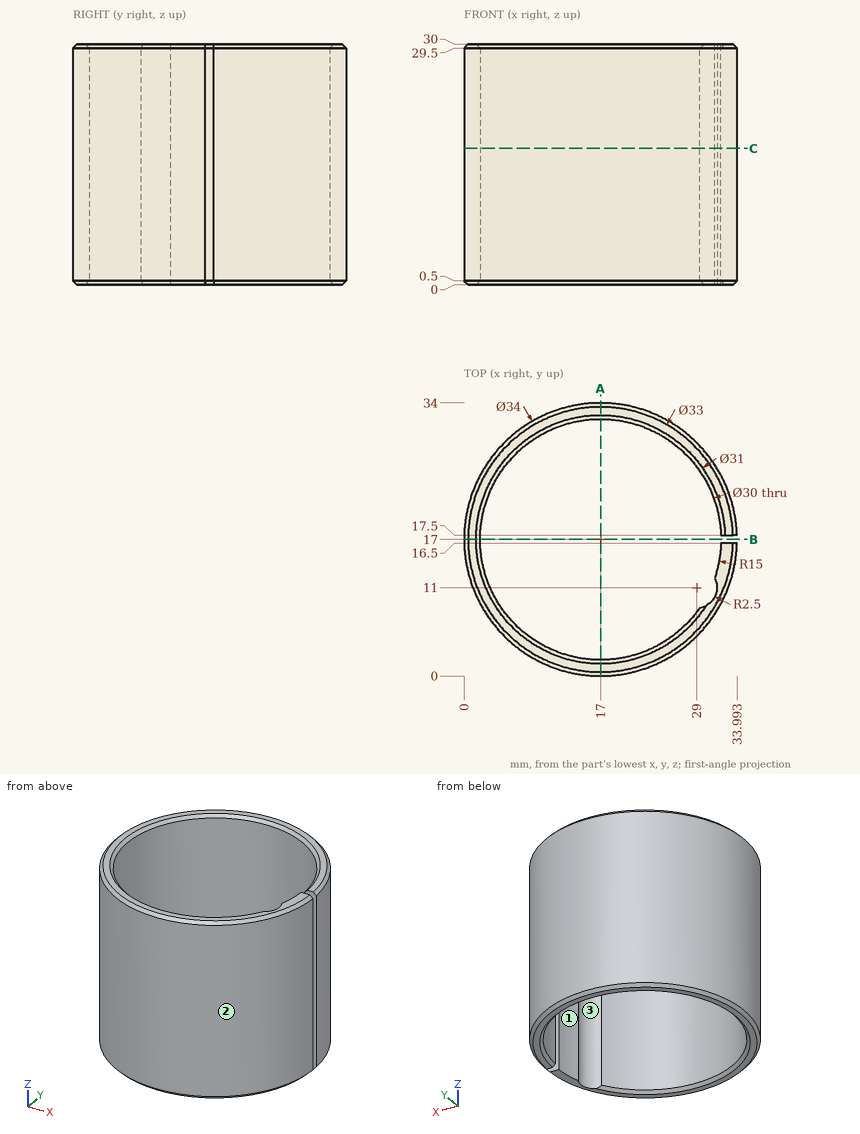
Part print with two shaded views. Sizes in mm from the minimum x, y, z corner. Round coordinates to 2 decimals unless told otherwise and drop trailing zeros. Order: outer loops, then holes, each group sorted by start corner. A loop starts at its lowest first (then second) coordinate and runs counter-clockwise, first axis right, second up.
(1) Pin check, flat tips, straight feed: pin 1 (2 mm diameter, centred on x = 20.5, z = 9.5, fed in from +Y) (1 decimal); pin 2 (1.6 mm diameter, centred on x = 33.5, z = 19.5, fed in from -Y); pin 3 (6 mm diameter, centred on x = 9, z = 17.5, fed in from +Y). Stop position of each tip, or through.
(2) Band-saw the part on C-C (z = 17). List the corners of the cut face in (x, y) (1 decimal).
(3) Band-saw the part on A-A (x = 17). List the corners of the cut face in (y, z), then the cut area to 3 significant figures.
(4) Drill centre lines: line 1 (Y direction, x = 17, z = 19.75); line 2 (Y direction, x = 21, z = 16.5); line 3 (X direction, y = 19.5, z = 17.5) (1 decimal). Where is each one in solid material? Low to high.
(5) Pull direction Y, two halves, no side cores. Call the marked faces 1, 2 and 3: released by +Y, released by -Y, zero draft, split by the parting line, or undercut.
(6) Band-saw the part on B-B (y = 17). List the corners of the cut face in (x, z).
Verdict:
1. pin 1: stops at y = 33.8
1. pin 2: stops at y = 10.48
1. pin 3: stops at y = 33.25
2. outline: (29.4, 8.5) arc R15 cw (long way) to (32, 17.5) - (34, 17.5) arc R17 ccw (long way) to (34, 16.5) - (32, 16.5) arc R15 cw to (31.2, 12.2) arc R2.5 cw to start
3. outline: (0, 0.5) - (0.5, 0) - (1.5, 0) - (2, 0.5) - (2, 29.5) - (1.5, 30) - (0.5, 30) - (0, 29.5) - close; (32, 0.5) - (32.5, 0) - (33.5, 0) - (34, 0.5) - (34, 29.5) - (33.5, 30) - (32.5, 30) - (32, 29.5) - close
3. area: 119 mm2
4. line 1: y = 0 to 2, 32 to 34
4. line 2: y = 0.48 to 2.54, 31.46 to 33.52
4. line 3: x = 0.2 to 2.2, 31.8 to 33.8
5. face 1: undercut
5. face 2: split by the parting line
5. face 3: undercut
6. outline: (0, 0.5) - (0.5, 0) - (1.5, 0) - (2, 0.5) - (2, 29.5) - (1.5, 30) - (0.5, 30) - (0, 29.5) - close
